from build123d import *

# Parameters (mm, degrees)
F1_DEPTH = 63.5
F2_DEPTH = 25.4
F0_W     = 37.3578295112
F0_H     = 13.7197794846
F0_H_2   = 23.6380351254
F0_H_3   = 11.7702707648
F3_DEPTH = 28.575


with BuildPart() as f1:
    # F0 (on Front) → F1 (new body, symmetric)
    with BuildSketch(Plane.XZ):
        Polygon((35.526488953, 20.0833715498), (-59.1645240784, 20.0833715498), (-59.1645240784, -20.0833715498), (59.1645240784, -20.0833715498), (59.1645240784, 20.0833715498), align=None)
    extrude(amount=F1_DEPTH, both=True)

    # F0 (on Front) → F2 (join, symmetric)
    with BuildSketch(Plane.XZ):
        with BuildLine():
            Line((35.526488953, 76.3945057988), (35.526488953, 20.0833715498))
            Line((35.526488953, 20.0833715498), (59.1645240784, 20.0833715498))
            Line((59.1645240784, 20.0833715498), (59.1645240784, 76.3945057988))
            ThreePointArc((59.1645240784, 76.3945057988), (64.2012826279, 87.7945426192), (76.0210826993, 91.7470231652))
            Line((76.0210826993, 91.7470231652), (104.1673794389, 91.7470231652))
            Line((104.1673794389, 91.7470231652), (104.1673794389, 115.3850582906))
            Line((104.1673794389, 115.3850582906), (76.8725928536, 115.3850582906))
            add(Edge.make_bspline(
                [(66.1712992482, 114.5353537972), (69.7326775282, 114.9157218144), (73.3029348697, 115.1988448631), (76.8725928536, 115.3850582906)],
                knots=[156.3347304478, 156.3347304478, 156.3347304478, 156.3347304478, 166.0978888451, 166.0978888451, 166.0978888451, 166.0978888451], degree=3))
            ThreePointArc((66.1712992482, 114.5353537972), (44.1367599152, 100.8578900908), (35.526488953, 76.3945057988))
        make_face()
    extrude(amount=F2_DEPTH, both=True)

    # F0 (on Front) → F3 (join, symmetric)
    with BuildSketch(Plane.XZ):
        with Locations((122.8462941945, 122.2449480329)):
            Rectangle(F0_W, F0_H)
        with Locations((122.8462941945, 103.5660407279)):
            Rectangle(F0_W, F0_H_2)
        with Locations((122.8462941945, 85.8618877828)):
            Rectangle(F0_W, F0_H_3)
        Polygon((141.52520895, 129.1048377752), (141.52520895, 115.3850582906), (141.52520895, 91.7470231652), (141.52520895, 79.9767524004), (178.8830384612, 79.9767524004), (178.8830384612, 129.1048377752), align=None)
    extrude(amount=F3_DEPTH, both=True)


solid = f1.part
Here's how the part is built. I have some questions about the finished solid (model axes, mm). A direction names the side the tool comes from. Give positions to 0.01 mm unless a question says otherwise; leave off trailing zeros. Loops run counter-clockwise (first coordinate to the right, second up) from the corner with the lowest first, then second, coordinate; pieces in that order, holes last. Notation, with made-up numbers: (-15, -34) -> (-8, -34) arc R25 ccw to (-8, 5) -> close; hole circle Ø10 at (-28, 24). An arc over 180 degrees is marked (long way). One line per item, written item: value.
Q1. Suppose I cut it at C-C on z = 4. Please give me the cut outline in (x, y).
Answers follow:
outline: (-59.16, -63.5) -> (59.16, -63.5) -> (59.16, 63.5) -> (-59.16, 63.5) -> close
Q2. Suppose I cut it at B-B on x = 53. Please give me the cut outline in (y, z), then the cut area to 3 significant figures.
Answers follow:
outline: (-63.5, -20.08) -> (63.5, -20.08) -> (63.5, 20.08) -> (25.4, 20.08) -> (25.4, 108.95) -> (-25.4, 108.95) -> (-25.4, 20.08) -> (-63.5, 20.08) -> close
area: 9,620 mm^2
Q3. If I drill on line 1 along Z through (x, y) = (23.5, -20.5); line 2 along X through (y, z) = (11, 75); line 3 along X through (y, z) = (58, 12), over which ranges is the centre line in solid material (lowest first)?
Answers follow:
line 1: -20.08 to 20.08
line 2: 35.53 to 59.16
line 3: -59.16 to 59.16
Q4. Suppose I cut it at D-D on y = -36. Please give me the cut outline in (x, z).
Answers follow:
outline: (-59.16, -20.08) -> (59.16, -20.08) -> (59.16, 20.08) -> (-59.16, 20.08) -> close
Q5. On a 3-axis mill with a long thin cutter (end or side, diameter ignored), from which of +Z, -Z, +X, -X, +Y, -Y can I reach the whole of each face in a straight line? I mean faces 1 (the face through (141, 0, 79.977)), 2 (the face through (90, 0, 91.747)), 3 (the face through (91, 0, 115.385)), 4 (the face through (54, 25.4, 79)). Say none if no direction works.
Answers follow:
face 1: -Z, +X, +Y, -Y
face 2: -Z, +Y, -Y
face 3: +Z, -X, +Y, -Y
face 4: +Z, -X, +Y
Q6. Suppose I cut it at A-A on z = 86.5. Please give me the cut outline in (x, y) (3 decimals), then the cut area to 3 significant figures.
Answers follow:
outline: (36.856, -25.4) -> (62.938, -25.4) -> (62.938, 25.4) -> (36.856, 25.4) -> close; (104.167, -28.575) -> (178.883, -28.575) -> (178.883, 28.575) -> (104.167, 28.575) -> close
area: 5,590 mm^2
Q7. I'm going to push flat-ended pins straight in: pin 1 Ø1.5 at (x, y) = (130.5, 21) entering from -Z; pin 2 Ø5 at (x, y) = (-10.5, 16.5) entering from +Z; pin 3 Ø1.5 at (y, z) = (-5, 78) entering from +X. Where does each tip first touch, or does it pass through?
Answers follow:
pin 1: z = 79.98
pin 2: z = 20.08
pin 3: x = 59.35
Q8. We'd pull the mould along X, two halves only. Please class faces 5 (the face through (-1, -1, -20.083)), 6 (the face through (44.37, -0.356, 101.145)), 7 (the face through (104.167, 0, 116)), 8 (the face through (64.1, -0.4, 87.7)): pulls with the +X half, pulls with the -X half, needs draft (parallel to the pull), parting line crosses it, or undercut.
Answers follow:
face 5: needs draft
face 6: pulls with the -X half
face 7: undercut
face 8: undercut
